Can you work these out from the model? Positions are in its coordinate system, mm. A direction names the side the tool comes from. Round coordinates to 2 decimals unless told otherwise and drop trailing zeros. Write each loop counter-clockwise with the first axis right and the second up, starting at its lowest first coordinate (ties: lowest second). Pieces come first, ordered by that corner, then holes. Notation, with made-up numbers: M 8.5,12 L 62.5,12 A7 cw 62.5,22 Z; hole C -13,56.5 d11. An arc over 180 degrees is marked long. Answer as a JSON object with one key per item and string values. Group by question number.
1) If we mould it in two halves opening along Z, with no side actions, what happens to faces 1 (the cylindrical face through (6.37, -18.96, 40.5)), 2 (the cylindrical face through (6.26, -11.2, 27.52)), 3 (the flat face through (37.351, -8.576, 27.29))? For each: +Z half, -Z half, draft (parallel to the pull), parting line (faces both ways), or undercut.
2) On a 3-axis mill with a long thin cutter (end or side, diameter ignored), from which of +Z, -Z, +X, -X, +Y, -Y can I reach the whole of each face in a straight line? I mean faces 4 (the flat face through (37.351, -13.547, 23.674)), 5 (the flat face through (43.24, -6.033, 39.402)), 6 (the flat face through (10, -0.867, 40)), 7 (the flat face through (37.351, -8.318, 61.127)). Say none if no direction works.
3) Suppose I cut it at B-B, the plane y = 2. Write out the boundary of the cut face in (x, z), and give its area (3 significant figures).
4) Suppose I cut it at A-A, the plane z = 16. Write out the boundary of the cut face in (x, y).
5) Suppose I cut it at D-D, the plane x = 41. Write out the boundary of the cut face in (y, z).
6) Suppose I cut it at C-C, the plane z = 59.5. Write out the boundary of the cut face in (x, y).
7) Please list where these lines run through material, in increasing order: L1, parallel to Y at x = 4, z = 60 (3 decimals); L2, parallel to Z at x = 1, y = 0; L3, parallel to Z at x = 31.5, y = -8. Write a range as [from, to].
8) I'm going to push flat-ended pins straight in: pin 1 Ø4 at (y, z) = (-7.5, 60) entering from -X; pin 2 Ø4 at (x, z) = (24.5, 28) entering from +Y; pin 3 Ø4 at (x, z) = (1.5, 47) entering from +Y; pin 4 Ø10 at (y, z) = (-17, 14) entering from +X. Where does each tip first touch, or does it pass through?
from build123d import *

# Parameters (mm, degrees)
F0_W           = 42.9559741169
F0_H           = 39.4349899143
F1_DEPTH       = 42.672
F3_D           = 12.7
F3_DEPTH       = 50.8
F3_TIP         = 3.8154649308
F5_D           = 12.7
F5_CBORE_D     = 15.24
F5_CBORE_DEPTH = 19.05
F6_SIZE        = 5.08
F7_T1_DEPTH    = 54.102
F7_T3_DEPTH    = 49.3059741169
F7_T5_DEPTH    = 24.1949899143
F7_S9_W        = 7.62
F7_S9_H        = 7.62
F7_T10_DEPTH   = 7.62
F7_S15_W       = 7.62
F7_S15_H       = 7.62
F7_T16_DEPTH   = 7.62
F11_R          = 7.1053142902
F12_DEPTH      = 25.9
F14_DEPTH      = 26.5
F15_DEPTH      = 29.3
F16_R          = 4.5
F17_DEPTH      = 25
F18_R          = 7.4357269109
F19_DEPTH      = 25


# Not quite as in the source:
# - a fillet or chamfer that OpenCascade refuses, or shapes differently, is made with other operations: its cross-section is extruded or revolved along the edge and cut away or added
# - the program builds the solid bodies; features that only make, move or delete a surface that nothing else refers to are left out


with BuildPart() as f1:
    # F0 (on Top) → F1 (new body)
    with BuildSketch(Plane.XY):
        with Locations((2.8086053208, -1.5343176201)):
            Rectangle(F0_W, F0_H)
    extrude(amount=F1_DEPTH)

    # F3
    with Locations(Plane.YZ.offset(24.2865923792)):
        with Locations((0, 21.336)):
            Hole(F3_D / 2, depth=F3_DEPTH)
            with Locations((0, 0, -(F3_DEPTH + F3_TIP / 2))):  # 118° drill point
                Cone(0, F3_D / 2, F3_TIP, mode=Mode.SUBTRACT)

    # F5 (through all)
    with Locations(Plane(origin=(0, 18.1831773371, 0), x_dir=(-1, 0, 0), z_dir=(0, 1, 0))):
        with Locations((-7.6360311359, 33.7194018066)):
            CounterBoreHole(F5_D / 2, F5_CBORE_D / 2, F5_CBORE_DEPTH)

    # F6
    f6_edges = [f1.edges().sort_by_distance(p)[0] for p in [
        (24.286592, -1.534318, 42.672),
    ]]
    chamfer(f6_edges, length=F6_SIZE)

    # F7: fillet of radius 7.62 on 5 edges, made by hand

    # F7_s2 → F7_t1 (cut)
    with BuildSketch(Plane.XY.offset(-19.05)):
        with BuildLine():
            ThreePointArc((-11.0493817377, 18.1831773371), (-16.4375354104, 15.9513310097), (-18.6693817377, 10.5631773371))
            Line((-18.6693817377, 10.5631773371), (-18.6693817377, 18.1831773371))
            Line((-18.6693817377, 18.1831773371), (-11.0493817377, 18.1831773371))
        make_face()
        with BuildLine():
            ThreePointArc((-18.6693817377, -13.6318125772), (-16.4375354104, -19.0199662499), (-11.0493817377, -21.2518125772))
            Line((-11.0493817377, -21.2518125772), (-18.6693817377, -21.2518125772))
            Line((-18.6693817377, -21.2518125772), (-18.6693817377, -13.6318125772))
        make_face()
    extrude(amount=F7_T1_DEPTH, mode=Mode.SUBTRACT)

    # F7_s4 → F7_t3 (cut)
    with BuildSketch(Plane.YZ.offset(-11.0493817377)):
        with BuildLine():
            ThreePointArc((18.1831773371, 35.052), (15.9513310097, 40.4401536726), (10.5631773371, 42.672))
            Line((10.5631773371, 42.672), (18.1831773371, 42.672))
            Line((18.1831773371, 42.672), (18.1831773371, 35.052))
        make_face()
        with BuildLine():
            ThreePointArc((-13.6318125772, 42.672), (-19.0199662499, 40.4401536726), (-21.2518125772, 35.052))
            Line((-21.2518125772, 35.052), (-21.2518125772, 42.672))
            Line((-21.2518125772, 42.672), (-13.6318125772, 42.672))
        make_face()
    extrude(amount=F7_T3_DEPTH, mode=Mode.SUBTRACT)

    # F7_s6 → F7_t5 (cut)
    with BuildSketch(Plane.XZ.offset(-10.5631773371)):
        with BuildLine():
            ThreePointArc((-11.0493817377, 42.672), (-16.4375354104, 40.4401536726), (-18.6693817377, 35.052))
            Line((-18.6693817377, 35.052), (-18.6693817377, 42.672))
            Line((-18.6693817377, 42.672), (-11.0493817377, 42.672))
        make_face()
    extrude(amount=F7_T5_DEPTH, mode=Mode.SUBTRACT)


with BuildPart() as f7_tool8:
    # F7_s9 → F7_t10 (new body)
    with BuildSketch(Plane.XZ.offset(-10.5631773371)):
        with Locations((-14.8593817377, 38.862)):
            Rectangle(F7_S9_W, F7_S9_H)
    extrude(amount=-F7_T10_DEPTH)

    # F7_s11 → F7_t12 (revolve, cut)
    with BuildSketch(Plane(origin=(-11.0493817377, 10.5631773371, 35.052), x_dir=(0.7071067812, 0, -0.7071067812), z_dir=(0.7071067812, 0, 0.7071067812))):
        with BuildLine():
            ThreePointArc((0, -7.62), (7.62, 0), (0, 7.62))
            Line((0, 7.62), (0, -7.62))
        make_face()
    revolve(axis=Axis((-11.0493817377, 10.5631773371, 35.052), (0, 1, 0)), mode=Mode.SUBTRACT)


with BuildPart() as f1_1:
    add(f1.part)

    # F7_t7: cut F7_tool8
    add(f7_tool8.part, mode=Mode.SUBTRACT)


with BuildPart() as f7_tool14:
    # F7_s15 → F7_t16 (new body)
    with BuildSketch(Plane.XY.offset(35.052)):
        with Locations((-14.8593817377, -17.4418125772)):
            Rectangle(F7_S15_W, F7_S15_H)
    extrude(amount=F7_T16_DEPTH)

    # F7_s17 → F7_t18 (revolve, cut)
    with BuildSketch(Plane(origin=(-11.0493817377, -13.6318125772, 35.052), x_dir=(0.7071067812, 0.7071067812, 0), z_dir=(0.7071067812, -0.7071067812, 0))):
        with BuildLine():
            ThreePointArc((0, -7.62), (7.62, 0), (0, 7.62))
            Line((0, 7.62), (0, -7.62))
        make_face()
    revolve(axis=Axis((-11.0493817377, -13.6318125772, 35.052), (0, 0, 1)), mode=Mode.SUBTRACT)


with BuildPart() as f1_2:
    add(f1_1.part)

    # F7_t13: cut F7_tool14
    add(f7_tool14.part, mode=Mode.SUBTRACT)

    # F11 (on face) → F12 (join)
    with BuildSketch(Plane.XY.offset(42.672)):
        with Locations((4.0786053208, -1.5343176201)):
            Circle(F11_R)
    extrude(amount=F12_DEPTH)

    # F13 (on face) → F14 (join)
    with BuildSketch(Plane.YZ.offset(24.2865923792)):
        Polygon((-6.8631088361, 31.5118990839), (-16.0354040563, 32.4774049222), (-16.7595334351, 24.1499263793), (-10.2423755452, 23.1844205409), align=None)
    extrude(amount=F14_DEPTH)

    # F15 (add): a face of the model
    f15_faces = [f1_2.faces().sort_by_distance(p)[0] for p in [
        (37.5365923792, -11.4492564462, 31.994652003),
    ]]
    extrude(f15_faces, amount=F15_DEPTH)

    # F16 (on face) → F17 (cut)
    with BuildSketch(Plane.XY.offset(68.572)):
        with Locations((4.0786053208, -1.5343176201)):
            Circle(F16_R)
    extrude(amount=-F17_DEPTH, mode=Mode.SUBTRACT)

    # F18 (on face) → F19 (cut)
    with BuildSketch(Plane(origin=(0, -10.0685909657, 1.0598528644), x_dir=(-1, 0, 0), z_dir=(0, 0.9945054407, -0.1046849002))):
        with Locations((-37.5365923792, 45.2702912239)):
            Circle(F18_R)
    extrude(amount=-F19_DEPTH, mode=Mode.SUBTRACT)


solid = f1_2.part
Results:
{
 "1": {"face 1": "+Z half", "face 2": "undercut", "face 3": "-Z half"},
 "2": {"face 4": "-Z, +X, -Y", "face 5": "-Z, +X, +Y", "face 6": "+Y", "face 7": "+Z, +X, +Y"},
 "3": {"outline": "M -18.67,0 L 24.29,0 L 24.29,15.31 L -18.67,15.31 Z; M -18.67,27.36 L 3.43,27.36 A7.62 cw long 11.84,27.36 L 24.29,27.36 L 24.29,37.59 L 19.21,42.67 L 10.24,42.67 L 10.24,68.57 L 6.86,68.57 L 6.86,43.57 L 1.29,43.57 L 1.29,68.57 L -2.09,68.57 L -2.09,42.67 L -11.05,42.67 A7.62 ccw -18.67,35.05 Z", "area": "1,290 mm^2"},
 "4": {"outline": "M -18.67,-13.63 A7.62 ccw -11.05,-21.25 L 24.29,-21.25 L 24.29,-3.44 L -18.67,-3.44 Z; M -18.67,3.44 L 24.29,3.44 L 24.29,18.18 L -11.05,18.18 A7.62 ccw -18.67,10.56 Z"},
 "5": {"outline": "M -16.76,24.15 L -10.24,23.18 L -6.86,31.51 L -6.02,39.54 L -15.19,40.5 L -16.04,32.48 Z; M -13.81,53.59 L -4.64,52.63 L -3.8,60.65 L -12.97,61.62 Z"},
 "6": {"outline": "C 4.08,-1.53 d14.21; M 24.29,-13.19 L 50.79,-13.19 L 50.79,-3.92 L 24.29,-3.92 Z; hole C 4.08,-1.53 d9"},
 "7": {"L1": "[-8.639, -6.034], [2.965, 5.571]", "L2": "[0, 14.99], [27.69, 29.97], [37.46, 43.57]", "L3": "[28.71, 42], [50.73, 61.09]"},
 "8": {"pin 1": "x = -1.82", "pin 2": "y = 18.18", "pin 3": "y = 5.55", "pin 4": "x = 24.29"}
}
